```python
from build123d import *

# Parameters (mm, degrees)
SKETCH1_R           = 1.65
BOSS_EXTRUDE1_DEPTH = 15
CUT_EXTRUDE1_DEPTH  = 10
FILLET1_R           = 8
CUT_EXTRUDE2_DEPTH  = 11
SKETCH4_R           = 2.1
CUT_EXTRUDE3_DEPTH  = 3.5
FILLET2_R           = 5
FILLET3_R           = 20
FILLET5_R           = 1


with BuildPart() as part:
    # Sketch1 → Boss-Extrude1 (new body, symmetric)
    with BuildSketch(Plane.XY):
        with BuildLine():
            Line((0, 5), (-40, 5))
            Line((-40, 5), (-40, -5))
            Line((-40, -5), (0, -5))
            ThreePointArc((0, -5), (5, 0), (0, 5))
        make_face()
        Circle(SKETCH1_R, mode=Mode.SUBTRACT)
    extrude(amount=BOSS_EXTRUDE1_DEPTH, both=True)

    # Sketch2 → Cut-Extrude1 (cut, symmetric)
    with BuildSketch(Plane.XY):
        with BuildLine():
            Line((-5, 5), (0, 5))
            ThreePointArc((0, 5), (5, 0), (0, -5))
            Line((0, -5), (-5, -5))
            Line((-5, -5), (-5, 5))
        make_face()
    extrude(amount=CUT_EXTRUDE1_DEPTH, both=True, mode=Mode.SUBTRACT)

    # Fillet1
    fillet1_edges = [part.edges().sort_by_distance(p)[0] for p in [
        (-5, -5, 0),
    ]]
    fillet(fillet1_edges, radius=FILLET1_R)

    # Sketch3 → Cut-Extrude2 (cut, through all)
    with BuildSketch(Plane.XZ.offset(5)):
        Polygon((-40, 8.75), (-30, 8.75), (-13, 15), (-40, 15), align=None)
        Polygon((-13, -15), (-40, -15), (-40, -8.75), (-30, -8.75), align=None)
    extrude(amount=-CUT_EXTRUDE2_DEPTH, mode=Mode.SUBTRACT)

    # Sketch4 → Cut-Extrude3 (cut)
    with BuildSketch(Plane(origin=(0, 5, 0), x_dir=(1, 0, 0), z_dir=(0, 1, 0))):
        with Locations((-35, 5)):
            Circle(SKETCH4_R)
        with Locations((-35, -5)):
            Circle(SKETCH4_R)
    cut_extrude3 = extrude(amount=-CUT_EXTRUDE3_DEPTH, mode=Mode.SUBTRACT)

    # Fillet2
    fillet2_edges = [part.edges().sort_by_distance(p)[0] for p in [
        (-40, 0, 8.75),
        (-40, 0, -8.75),
    ]]
    fillet(fillet2_edges, radius=FILLET2_R)

    # Fillet3
    fillet3_edges = [part.edges().sort_by_distance(p)[0] for p in [
        (-13, 0, 15),
        (-30, 0, 8.75),
        (-30, 0, -8.75),
        (-13, 0, -15),
    ]]
    fillet(fillet3_edges, radius=FILLET3_R)

    # Fillet5
    fillet5_edges = [part.edges().sort_by_distance(p)[0] for p in [
        (-34.279993099, -5, 8.75),
        (-34.279993099, 5, 8.75),
        (-40, -5, 0),
        (-38.535533906, -5, -7.285533906),
        (-38.535533906, -5, 7.285533906),
        (-40, 5, 0),
        (-38.535533906, 5, -7.285533906),
        (-38.535533906, 5, 7.285533906),
        (-21.5, -5, -11.875),
        (-21.5, 5, -11.875),
        (-34.279993099, -5, -8.75),
        (-4.720006901, -5, -15),
        (-4.720006901, -5, 15),
        (-21.5, -5, 11.875),
        (-12.944908854, -5, 14.690497979),
        (-12.944908854, -5, -14.690497979),
        (-21.5, 5, 11.875),
        (-34.279993099, 5, -8.75),
        (-12.944908854, 5, 14.690497979),
        (-12.944908854, 5, -14.690497979),
        (-30.055091146, -5, -9.059502021),
        (-30.055091146, 5, -9.059502021),
        (-30.055091146, -5, 9.059502021),
        (-30.055091146, 5, 9.059502021),
        (5, 0, 15),
        (-4.720006901, 5, -15),
        (5, 0, -15),
        (-4.720006901, 5, 15),
    ]]
    fillet(fillet5_edges, radius=FILLET5_R)

    # Mirror1: Cut-Extrude3 across plane
    add(cut_extrude3.mirror(Plane.ZX), mode=Mode.SUBTRACT)


solid = part.part
```
Work out the finished part from the listing and answer in its coordinate system (mm). A direction names the side the tool comes from. Give positions to 0.01 mm unless a question says otherwise; leave off trailing zeros. Loops run counter-clockwise (first coordinate to the right, second up) from the corner with the lowest first, then second, coordinate; pieces in that order, holes last. Notation, with made-up numbers: (1.25, 86.5) -> (30.25, 86.5) arc R17 cw to (30.25, 107.5) -> close; hole circle Ø8 at (-21.5, -31.5). An arc over 180 degrees is marked (long way). Put each result on its own line as item: value. Start each with the question number.
Item 1: Each of these flat-tipped pins is pushed along its axis until it touches: P1, Ø2.5, axis at x = 0, y = 0, coming from the -Z side; P2, Ø6.5, axis at x = -35, z = -5, coming from the -Y side; P3, Ø2.5, axis at x = -35, z = 5, coming from the -Y side; P4, Ø2, axis at x = -35, z = 5, coming from the +Y side. Where does it stop, or does it pass through?
Item 2: The part is cut by section B-B (z = -1). Give the vertices of the cut face in (x, y).
Item 3: Which of the six approach directions +Z, -Z, +X, -X, +Y, -Y give full straight-line access (tool end or side, diameter ignored) to faces 4 (the face through (-34, 0, -8.75)), 5 (the face through (-34, 0, 8.75)), 6 (the face through (-37.1, 3.27, -5.09))?
Item 4: The part is cut by section C-C (y = -2.25). State how many separate pieces and enclosed holes the cut face has, then the cut area to 3 significant figures.
Item 5: The part is cut by section A-A (y = 0). Give the vertices of the cut face in (x, z).
Item 6: The mould has two halves that part along X. Classify faces 1 (the face through (-21.57, -0.06, -11.85)), 2 (the face through (-34.27, 4.699, -8.465)), 3 (the face through (-37.1, 3.27, 4.91)): released by +X, released by -X, zero draft, split by the parting line, or undercut.
Item 7: Find the intervals of material crossed by L1, parallel to Z at x = -35, y = -3.9; L2, parallel to Z at x = -2.5, y = -1.75; L3, parallel to Y at x = 0, z = -13, in increasing order. Write a range as [from, to].
Answers below:
1. P1: through
1. P2: y = -5
1. P3: y = -1.5
1. P4: y = 1.5
2. outline: (-40, -4) arc R1 ccw to (-39, -5) -> (-13, -5) arc R8 ccw to (-5, 3) -> (-5, 5) -> (-39, 5) arc R1 ccw to (-40, 4) -> close
3. face 4: -Z, -X, +Y, -Y
3. face 5: +Z, -X, +Y, -Y
3. face 6: +Y
4. separate pieces: 1
4. enclosed holes: 2
4. area: 835 mm2
5. outline: (-40, -3.75) arc R5 ccw to (-35, -8.75) -> (-33.56, -8.75) arc R20 cw to (-26.66, -9.98) -> (-16.34, -13.77) arc R20 ccw to (-9.44, -15) -> (-1.65, -15) -> (-1.65, -10) -> (-5.58, -10) -> (-5.58, 10) -> (-1.65, 10) -> (-1.65, 15) -> (-9.44, 15) arc R20 ccw to (-16.34, 13.77) -> (-26.66, 9.98) arc R20 cw to (-33.56, 8.75) -> (-35, 8.75) arc R5 ccw to (-40, 3.75) -> close; (1.65, -15) -> (4, -15) arc R1 ccw to (5, -14) -> (5, -10) -> (1.65, -10) -> close; (1.65, 10) -> (5, 10) -> (5, 14) arc R1 ccw to (4, 15) -> (1.65, 15) -> close
6. face 1: released by -X
6. face 2: zero draft
6. face 3: undercut
7. L1: [-8.75, -7.1], [-2.9, 2.9], [7.1, 8.75]
7. L2: [-15, -10], [10, 15]
7. L3: [-5, -1.65], [1.65, 5]
